Check sheet for the modelled part. Datum: model origin and axes. Units: mm. A direction names the side the tool comes from. Round coordinates to 2 decimals unless told otherwise and drop trailing zeros. Write each loop counter-clockwise with the first axis right and the second up, starting at its lowest first coordinate (ties: lowest second). Pieces come first, ordered by that corner, then holes. Notation, with made-up numbers: (84, 36) -> (124, 36) arc R24 ccw to (124, 50) -> close; hole circle Ø4 at (27, -3.5). An arc over 180 degrees is marked (long way). One line per item, written item: value.
from build123d import *

# Parameters (mm, degrees)
F0_W     = 3.8772569518
F0_H     = 63.9679611865
F0_W_2   = 3.5099290236
F1_DEPTH = 50.8


with BuildPart() as f1:
    # F0 (on Front) → F1 (new body)
    with BuildSketch(Plane.XZ):
        with Locations((-14.058026042, -9.1675467221)):
            Rectangle(F0_W, F0_H)
        Polygon((3.0713511857, 50.9821392888), (-15.9966545179, 22.8164338711), (-12.1193975661, 22.8164338711), (18.9136061812, 22.8164338711), (22.4235352048, 22.8164338711), align=None)
        Polygon((-12.1193975661, -41.1515273154), (-15.9966545179, -41.1515273154), (-15.9966545179, -44.7443164885), (22.7297032942, -44.7443164885), (22.4235352048, -41.1515273154), (18.9136061812, -41.1515273154), align=None)
        with Locations((20.668570693, -9.1675467221)):
            Rectangle(F0_W_2, F0_H)
    extrude(amount=F1_DEPTH)


solid = f1.part
Item 1: Depth check by flat-ended pin: pin 1 (12 mm diameter, centred on x = 13, y = -43.5, fed in from +Z); pin 2 (10 mm diameter, centred on x = -8.5, y = -38.5, fed in from +Z); pin 3 (1 mm diameter, centred on x = -2, y = -15.5, fed in from +Z). Enter the tip coordinate at first touch or a pass-through.
Result set:
pin 1: z = 45.26
pin 2: z = 41.28
pin 3: z = 44.23
Item 2: Material ranges on line 1 along X through (y, z) = (-21.5, 11.5); line 2 along Z through (x, y) = (-1, -45); line 3 along Z through (x, y) = (-10, -2), recorded low to high.
Result set:
line 1: -16 to -12.12, 18.91 to 22.42
line 2: -44.74 to -41.15, 22.82 to 44.97
line 3: -44.74 to -41.15, 22.82 to 31.67
Item 3: Release check for a two-part mould opening along X. For faces 1 (the flat face through (3, -25, -44.744)), 2 (the flat face through (22.424, -25, -10)), 3 (the flat face through (4, -25, -41.152)) record: pulls with the +X half, pulls with the -X half, needs draft (parallel to the pull), parting line crosses it, or undercut.
Result set:
face 1: needs draft
face 2: pulls with the +X half
face 3: undercut
Item 4: Sectioned sample at C-C (y = -15.5). Enter the section's corners in (x, z).
Result set:
outline: (-16, -44.74) -> (22.73, -44.74) -> (22.42, -41.15) -> (22.42, 22.82) -> (3.07, 50.98) -> (-16, 22.82) -> close; hole (-12.12, -41.15) -> (18.91, -41.15) -> (18.91, 22.82) -> (-12.12, 22.82) -> close
Item 5: Tool access check on faces 4 (the flat face through (-15.997, -25, -10)), 5 (the flat face through (-12.119, -25, -10)). Record the directions out of +Z, -Z, +X, -X, +Y, -Y that give a thin tool (end or side, any length) a straight path to the whole face; none if there is none.
Result set:
face 4: +Z, -Z, -X, +Y, -Y
face 5: +Y, -Y
Item 6: Sectioned sample at D-D (z = 25). Enter the section's corners in (x, y), then the cut area to 3 significant figures.
Result set:
outline: (-14.52, -50.8) -> (20.92, -50.8) -> (20.92, 0) -> (-14.52, 0) -> close
area: 1,800 mm^2
Item 7: Sectioned sample at A-A (z = -39). Enter the section's corners in (x, y), then the cut area to 3 significant figures.
Result set:
outline: (-16, -50.8) -> (-12.12, -50.8) -> (-12.12, 0) -> (-16, 0) -> close; (18.91, -50.8) -> (22.42, -50.8) -> (22.42, 0) -> (18.91, 0) -> close
area: 375 mm^2
Item 8: Sectioned sample at B-B (x = 13.5). Enter the section's corners in (y, z).
Result set:
outline: (-50.8, -44.74) -> (0, -44.74) -> (0, -41.15) -> (-50.8, -41.15) -> close; (-50.8, 22.82) -> (0, 22.82) -> (0, 35.8) -> (-50.8, 35.8) -> close
